Read the model definition and answer for the solid it produces. Units are mm, in the model's axes. Face numbers are marked on the shaded views. A direction names the side the tool comes from. Give positions to 0.01 mm unless a question says otherwise; leave off trailing zeros. Write each loop counter-clockwise with the first axis right and the second up, starting at its lowest first coordinate (ties: lowest second). Pieces come first, ordered by that corner, then holes. Notation, with made-up numbers: (5, 18) -> (39, 18) arc R20 ccw to (39, 49) -> close; hole circle Ø11 at (58, -24). An arc over 180 degrees is marked (long way). Write item = value, one per line.
from build123d import *

# Parameters (mm, degrees)
SKETCH_W     = 12
SKETCH_H     = 12
PAD_DEPTH    = 6
SKETCH001_R  = 1.925
HOLE_DEPTH   = 6.001
SKETCH002_R  = 4
POCKET_DEPTH = 3
FILLET_R     = 3


with BuildPart() as part:
    # Sketch → Pad (new body)
    with BuildSketch(Plane.XY):
        with Locations((6, 6)):
            Rectangle(SKETCH_W, SKETCH_H)
    extrude(amount=PAD_DEPTH)

    # Sketch001 (on Face6 of Pad) → Hole (cut, through all)
    with BuildSketch(Plane.XY.offset(6)):
        with Locations((6, 6)):
            Circle(SKETCH001_R)
    extrude(amount=-HOLE_DEPTH, mode=Mode.SUBTRACT)

    # Sketch002 (on Face5 of Hole) → Pocket (cut)
    with BuildSketch(Plane.XY.offset(6)):
        with Locations((6, 6)):
            Circle(SKETCH002_R)
    extrude(amount=-POCKET_DEPTH, mode=Mode.SUBTRACT)

    # Fillet
    fillet_edges = [part.edges().sort_by_distance(p)[0] for p in [
        (0, 0, 3),
        (12, 0, 3),
        (12, 12, 3),
        (0, 12, 3),
    ]]
    fillet(fillet_edges, radius=FILLET_R)


solid = part.part
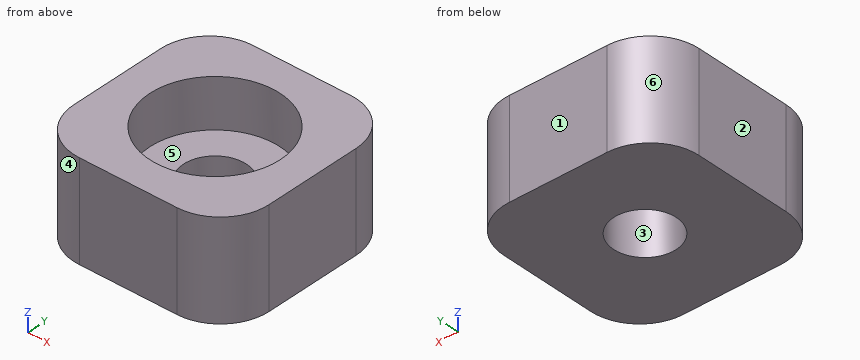
(1) A tool of negligible diameter and unlimited length cuts with its end or side. For the marked faces 5 and 6, from which of +Z, -Z, +X, -X, +Y, -Y can it reach the whole face along a straight path? Write none if from no direction.
Checks:
face_5 = +Z
face_6 = +Z, -Z, -X, +Y
(2) The part is cut by section D-D on x = 8.75. Determine the outline of the cut face in (y, z), plus the area to 3 significant figures.
Checks:
outline = (0, 0) -> (12, 0) -> (12, 6) -> (8.9, 6) -> (8.9, 3) -> (3.1, 3) -> (3.1, 6) -> (0, 6) -> close
area = 54.6 mm²
(3) Consider L1, parallel to Y at x = 6, z = 2.1 (3 decimals); L2, parallel to Y at x = 6, z = 4.7; L3, parallel to X at y = 7, z = 1.35. Determine where each line is inside the solid, lowest interval first.
Checks:
L1 = 0 to 4.075, 7.925 to 12
L2 = 0 to 2, 10 to 12
L3 = 0 to 4.36, 7.64 to 12
(4) The part is cut by section A-A on x = 6. Determine the outline of the cut face in (y, z) (3 decimals).
Checks:
outline = (0, 0) -> (4.075, 0) -> (4.075, 3) -> (2, 3) -> (2, 6) -> (0, 6) -> close; (7.925, 0) -> (12, 0) -> (12, 6) -> (10, 6) -> (10, 3) -> (7.925, 3) -> close
(5) For a pull along Y with two mould halves and no side action, classify the marked faces 1, 2, 3 and 4 as released by +Y, released by -Y, zero draft, split by the parting line, or undercut.
Checks:
face_1 = released by +Y
face_2 = zero draft
face_3 = undercut
face_4 = released by -Y
(6) The part is cut by section B-B on z = 1.6. Determine the outline of the cut face in (x, y) (3 decimals).
Checks:
outline = (0, 3) arc R3 ccw to (3, 0) -> (9, 0) arc R3 ccw to (12, 3) -> (12, 9) arc R3 ccw to (9, 12) -> (3, 12) arc R3 ccw to (0, 9) -> close; hole circle Ø3.85 at (6, 6)
(7) Given P1, Ø2, axis at x = 1.5, z = 4.5, coming from the -Y side; P2, Ø7, axis at x = 6, y = 6, coming from the +Z side; P3, Ø3, axis at x = 6, y = 6, coming from the +Z side, each flat-ended and moving along its own axis, determine where each tip first touches the part or whether it passes through.
Checks:
P1 = 0.04
P2 = 3
P3 = through
